from build123d import *

# Parameters (mm, degrees)
F0_R     = 2.54
F1_DEPTH = 15.24
F2_R     = 5.08
F3_R     = 2.54
F4_DEPTH = 15.748


with BuildPart() as f1:
    # F0 (on Front) → F1 (new body)
    with BuildSketch(Plane.XZ):
        Polygon((-26.816706221, 12.8465024581), (-26.816706221, -10.6672204749), (-26.816706221, -10.8938248026), (-17.7876478214, -33.9755966375), (8.7138581745, -23.6088168675), (49.6632434885, -23.6088168675), (49.6632434885, 0.9602710623), align=None)
        with Locations((-11.2967565115, -16.1095818214)):
            Circle(F0_R, mode=Mode.SUBTRACT)
        with Locations((3.9432434885, -12.1794487806)):
            Circle(F0_R, mode=Mode.SUBTRACT)
        with Locations((19.1832434885, -8.4152225918)):
            Circle(F0_R, mode=Mode.SUBTRACT)
        with Locations((34.4232434885, -5.1024009119)):
            Circle(F0_R, mode=Mode.SUBTRACT)
    extrude(amount=F1_DEPTH)

    # F2
    f2_edges = [f1.edges().sort_by_distance(p)[0] for p in [
        (-26.816706, -7.62, 12.846502),
        (49.663243, -7.62, 0.960271),
        (49.663243, -7.62, -23.608817),
        (8.713858, -7.62, -23.608817),
        (-17.787648, -7.62, -33.975597),
        (-26.816706, -7.62, -10.893825),
    ]]
    fillet(f2_edges, radius=F2_R)

    # F3 (on face) → F4 (cut)
    with BuildSketch(Plane(origin=(1.3170078158, 0, 8.474064501), x_dir=(0.988137358, 0, -0.1535726597), z_dir=(0.1535726597, 0, 0.988137358))):
        with Locations((32.3229017764, -7.62)):
            Circle(F3_R)
        with Locations((17.0829017764, -7.62)):
            Circle(F3_R)
        with Locations((1.8429017764, -7.62)):
            Circle(F3_R)
        with Locations((-13.3970982236, -7.62)):
            Circle(F3_R)
    extrude(amount=-F4_DEPTH, mode=Mode.SUBTRACT)


solid = f1.part
Source: CAD feature listing. Evaluate the final solid. Frame: model axes, mm. A direction names the side the tool comes from. Round coordinates to 2 decimals unless told otherwise and drop trailing zeros. Loops run counter-clockwise (first coordinate to the right, second up) from the corner with the lowest first, then second, coordinate; pieces in that order, holes last. Notation, with made-up numbers: (79.5, -3) - (103.5, -3) arc R36 ccw to (103.5, 36) - close; hole circle Ø11 at (-14, 8.25). An arc over 180 degrees is marked (long way). Write item = value, one per line. Start each with the question number.
Item 1: First-contact query: pin 1 Ø1.5 at (y, z) = (-6, -21.5) entering from +X; pin 2 Ø5 at (y, z) = (-8, 2.5) entering from +X; pin 3 Ø4.5 at (x, y) = (20, -9) entering from -Z. Flat tips, straight axial feed; report the tip coordinate or a pass-through.
Item 2: Section query A-A on z = -17.5. Output: boundary loops of the cut face in (x, y), plus the area to 3 significant figures.
Item 3: Mould query, pull axis Y, two halves, no side actions, for faces 1 (the face through (2, 0, -10)), 2 (the face through (-14.375, -7.584, -5.024)), 3 (the face through (3.61, -7.51, -9.66)), 4 (the face through (-13.44, -5.1, 2.91)). Classes: released by +Y, released by -Y, zero draft, split by the parting line, or undercut.
Item 4: Section query C-C on x = 23.5. Output: boundary loops of the cut face in (y, z), plus the area to 3 significant figures.
Item 5: Section query D-D on z = -22.5. Output: boundary loops of the cut face in (x, y).
Item 6: Section query B-B on y = -12. Output: boundary loops of the cut face in (x, z).
Item 7: Material intervals for line 1 (X direction, y = -4.5, z = -5); line 2 (X direction, y = -7, z = -17.5); line 3 (Z direction, x = -13.5, y = -12.5), sorted ascending.
Item 8: Reachability of faces 5 (the face through (-26.817, -8, -1)), 6 (the face through (27, -8, -23.609)), 7 (the face through (30.803, -7.584, -12.046)) from +Z, -Z, +X, -X, +Y, -Y: full face, straight path, thin tool, end or side. Return the list, or none.
Results list:
q1.pin_1 = 49.15
q1.pin_2 = 48.37
q1.pin_3 = -23.61
q2.outline = (-24.23, -15.24) - (-13.42, -15.24) - (-13.42, 0) - (-24.23, 0) - close; (-9.17, -15.24) - (49.66, -15.24) - (49.66, 0) - (-9.17, 0) - close
q2.area = 1,060 mm²
q3.face_1 = released by +Y
q3.face_2 = undercut
q3.face_3 = zero draft
q3.face_4 = undercut
q4.outline = (-15.24, -23.61) - (0, -23.61) - (0, 5.03) - (-15.24, 5.03) - close
q4.area = 436 mm²
q5.outline = (-22.28, -15.24) - (47.75, -15.24) - (47.75, 0) - (-22.28, 0) - close
q6.outline = (-26.82, -9.94) arc R5.08 ccw to (-26.47, -11.79) - (-19.64, -29.24) arc R5.08 ccw to (-13.06, -32.12) - (7.82, -23.96) arc R5.08 cw to (9.67, -23.61) - (44.58, -23.61) arc R5.08 ccw to (49.66, -18.53) - (49.66, -3.39) arc R5.08 ccw to (45.36, 1.63) - (-20.96, 11.94) arc R5.08 ccw to (-26.82, 6.92) - close; hole circle Ø5.08 at (-11.3, -16.11); hole circle Ø5.08 at (3.94, -12.18); hole circle Ø5.08 at (19.18, -8.42); hole circle Ø5.08 at (34.42, -5.1)
q7.line_1 = -26.82 to 31.89, 36.96 to 49.66
q7.line_2 = -24.23 to -13.42, -9.17 to 49.66
q7.line_3 = -32.28 to -17.37, -14.85 to 10.78
q8.face_5 = +Z, -Z, -X, +Y, -Y
q8.face_6 = -Z, +X, +Y, -Y
q8.face_7 = none
